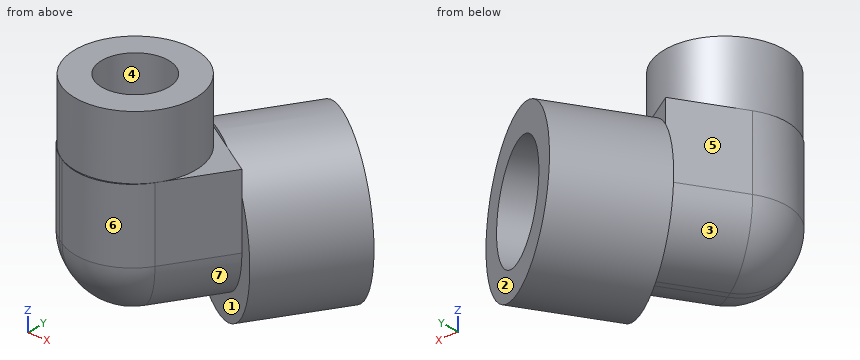
from build123d import *

# Parameters (mm, degrees)
CYLINDER021_R               = 5
CYLINDER021_DEPTH           = 25
CYLINDER022_R               = 5
CYLINDER022_DEPTH           = 15
CYLINDER020_R               = 9
CYLINDER020_DEPTH           = 9.5
BOX007_W                    = 19
BOX007_H                    = 18
BOX007_DEPTH                = 19.5
FILLET_R                    = 8.5
CYLINDER024_R               = 5
CYLINDER024_DEPTH           = 2.5
CYLINDER019_R               = 12
CYLINDER019_DEPTH           = 2.5
CYLINDER027_R               = 8
CYLINDER027_DEPTH           = 12.5
CYLINDER026_R               = 12
CYLINDER026_DEPTH           = 12.5
CYLINDER026_PLACEMENT_ANGLE = 1
FUSION025_PLACEMENT_ANGLE   = 90
FUSION042_ROLL_ANGLE        = 180
FUSION042_PLACEMENT_ANGLE   = 58.52


with BuildPart() as obj1_hole:
    # Cylinder021 → Cylinder021 (new body)
    with BuildSketch(Plane.XY):
        Circle(CYLINDER021_R)
    extrude(amount=CYLINDER021_DEPTH)


with BuildPart() as obj2:
    # Cylinder022 → Cylinder022 (new body)
    with BuildSketch(Plane(origin=(-5, 0, 21), x_dir=(0, 0, -1), z_dir=(1, 0, 0))):
        Circle(CYLINDER022_R)
    extrude(amount=CYLINDER022_DEPTH)

    # Fusion016: union obj1_hole
    add(obj1_hole.part)


with BuildPart() as obj1:
    # Cylinder020 → Cylinder020 (new body)
    with BuildSketch(Plane.XY):
        Circle(CYLINDER020_R)
    extrude(amount=CYLINDER020_DEPTH)


with BuildPart() as obj3:
    # Box007 → Box007 (new body)
    with BuildSketch(Plane(origin=(-9, -9, 9.5), x_dir=(1, 0, 0), z_dir=(0, 0, 1))):
        with Locations((9.5, 9)):
            Rectangle(BOX007_W, BOX007_H)
    extrude(amount=BOX007_DEPTH)

    # Fillet
    fillet_edges = [obj3.edges().sort_by_distance(p)[0] for p in [
        (-9, -9, 19.25),
        (-9, 0, 29),
        (-9, 9, 19.25),
        (0.5, -9, 29),
        (0.5, 9, 29),
    ]]
    fillet(fillet_edges, radius=FILLET_R)

    # Fusion018: union obj1
    add(obj1.part)

    # Cut013: cut obj2
    add(obj2.part, mode=Mode.SUBTRACT)


with BuildPart() as largeplughole:
    # Cylinder024 → Cylinder024 (new body)
    with BuildSketch(Plane.XY):
        Circle(CYLINDER024_R)
    extrude(amount=CYLINDER024_DEPTH)


with BuildPart() as largeplugbase001:
    # Cylinder019 → Cylinder019 (new body)
    with BuildSketch(Plane.XY):
        Circle(CYLINDER019_R)
    extrude(amount=CYLINDER019_DEPTH)

    # Cut008: cut LargePlugHole
    add(largeplughole.part, mode=Mode.SUBTRACT)


with BuildPart() as largeplugwallhole:
    # Cylinder027 → Cylinder027 (new body)
    with BuildSketch(Plane.XY.offset(2.5)):
        Circle(CYLINDER027_R)
    extrude(amount=CYLINDER027_DEPTH)


with BuildPart() as obj4:
    # Cylinder026 → Cylinder026 (new body)
    with BuildSketch(Plane.XY):
        Circle(CYLINDER026_R)
    extrude(amount=CYLINDER026_DEPTH)


with BuildPart() as obj4_1:
    # Cylinder026 placement: moved
    add(obj4.part.moved(Location((0, 0, 2.5))).rotate(Axis((0, 0, 2.5), (0, 0, 1)), CYLINDER026_PLACEMENT_ANGLE))

    # Cut007: cut LargePlugWallHole
    add(largeplugwallhole.part, mode=Mode.SUBTRACT)

    # Fusion025: union LargePlugBase001
    add(largeplugbase001.part)


with BuildPart() as obj4_2:
    # Fusion025 placement: moved
    add(obj4_1.part.moved(Location((10, 0, 21))).rotate(Axis((10, 0, 21), (0, 1, 0)), FUSION025_PLACEMENT_ANGLE))

    # Fusion042: union obj3
    add(obj3.part)


with BuildPart() as obj4_3:
    # Fusion042 roll: moved
    add(obj4_2.part.rotate(Axis((0, 0, 0), (1, 0, 0)), FUSION042_ROLL_ANGLE))


with BuildPart() as obj4_4:
    # Fusion042 placement: moved
    add(obj4_3.part.moved(Location((-39.5, -110, 63.5))).rotate(Axis((-39.5, -110, 63.5), (0, 0, 1)), FUSION042_PLACEMENT_ANGLE))


solid = obj4_4.part
Geometry: final body of the model. Coordinates: model frame, mm. Face numbers are marked on the shaded views. A direction names the side the tool comes from. Give positions to 0.01 mm unless a question says otherwise; leave off trailing zeros. Order: outer loops, then holes, each group sorted by start corner. A loop starts at its lowest first (then second) coordinate and runs counter-clockwise, first axis right, second up. Notation, with made-up numbers: (64, 86.25) -> (80, 86.25) arc R14 cw to (80, 95.25) -> close; hole circle Ø9 at (-27.75, 26). An arc over 180 degrees is marked (long way). Write each question's results on one line, items separated by ' | '.
1) Cut plane D-D (z = 34). Output: boundary loops of the cut face in (x, y).
Geometry says:
outline: (-41.5, -97.05) -> (-27.05, -105.9) -> (-19.22, -93.1) -> (-33.67, -84.26) -> close
2) Set-up query: the marked faces 4, 5, 6 and 7. Return all of +Z, -Z, +X, -X, +Y, -Y with unobstructed straight access to the full face (end or side cutting, diameter ignored); none if empty.
Geometry says:
face 4: +Z | face 5: +Z, -Z, -X | face 6: +Z, -Z, -Y | face 7: -Z, -Y
3) Cut plane A-A (z = 44). Output: boundary loops of the cut face in (x, y).
Geometry says:
outline: (-47.44, -105.73) arc R8.5 ccw to (-44.63, -117.41) -> (-43.77, -117.94) arc R8.5 ccw to (-32.09, -115.13) -> (-26.6, -106.17) -> (-24.12, -107.69) -> (-16.29, -94.9) -> (-19.74, -92.78) -> (-26.27, -103.44) -> (-28.9, -101.83) -> (-34.65, -111.21) arc R5 cw to (-36.22, -113.77) -> (-38.04, -116.75) -> (-46.18, -111.77) -> (-44.35, -108.79) arc R5 cw to (-42.78, -106.23) -> (-37.04, -96.85) -> (-39.67, -95.24) -> (-33.15, -84.58) -> (-36.6, -82.46) -> (-44.43, -95.25) -> (-41.95, -96.77) -> close
4) First-contact query: pin 1 Ø2 at (x, z) = (-32, 39) entering from +Y; pin 2 Ø1 at (x, y) = (-35, -107) entering from -Z; pin 3 Ø8 at (x, y) = (-35.5, -93) entering from +Z; pin 4 Ø5 at (x, y) = (-37.5, -113) entering from +Z. Flat tips, straight axial feed; report the tip coordinate or a pass-through.
Geometry says:
pin 1: stops at y = -84.67 | pin 2: stops at z = 34.6 | pin 3: stops at z = 54.41 | pin 4: stops at z = 63.5
5) Draft query along X for the marked faces 1, 2 and 3. Return one class per face: released by +X, released by -X, zero draft, split by the parting line, or undercut.
Geometry says:
face 1: undercut | face 2: released by +X | face 3: released by -X
6) Line query: line 1 along X through (y, z) = (-110, 59); line 2 along Y through (x, z) = (-39.5, 57.5); line 3 along Z through (x, y) = (-34, -88.5). Output: solid intervals per line, ascending.
Geometry says:
line 1: x = -48.5 to -44.5, -34.5 to -30.5 | line 2: y = -119 to -115, -105 to -101 | line 3: z = 32.44 to 37.89, 47.11 to 52.56
7) Cut plane B-B (z = 57.5). Output: boundary loops of the cut face in (x, y), and give its area (3 significant figures).
Geometry says:
outline: circle Ø18 at (-39.5, -110); hole circle Ø10 at (-39.5, -110) | area: 176 mm²
8) Cut plane C-C (z = 38). Output: boundary loops of the cut face in (x, y).
Geometry says:
outline: (-46.05, -106.58) arc R6.87 ccw to (-43.78, -116.03) -> (-42.92, -116.55) arc R6.87 ccw to (-33.47, -114.28) -> (-27.99, -105.32) -> (-24.79, -107.28) -> (-16.96, -94.49) -> (-20.8, -92.13) -> (-27.33, -102.79) -> (-31.11, -100.48) -> (-40.25, -115.4) -> (-43.97, -113.13) -> (-34.83, -98.2) -> (-38.61, -95.89) -> (-32.09, -85.23) -> (-35.93, -82.87) -> (-43.77, -95.66) -> (-40.57, -97.62) -> close
